from build123d import *

# Parameters (mm, degrees)
SKETCH_1_W                    = 120
SKETCH_1_H                    = 160
EXTRUDE_1_DEPTH               = 20
CHAMFER_1_SIZE                = 5
HOLE_WIZARD_M10_1_D           = 11
HOLE_WIZARD_M10_1_CBORE_D     = 18
HOLE_WIZARD_M10_1_CBORE_DEPTH = 10
CUT_EXTRUDE_1_REACH           = 103.98
SKETCH_6_R                    = 4


with BuildPart() as part:
    # 草圖1 → 伸長1 (new body)
    with BuildSketch(Plane(origin=(0, 0, 0), x_dir=(1, 0, 0), z_dir=(0, 1, 0))):
        Rectangle(SKETCH_1_W, SKETCH_1_H)
    extrude(amount=EXTRUDE_1_DEPTH)

    # 導角1
    chamfer_1_edges = [part.edges().sort_by_distance(p)[0] for p in [
        (-60, 10, -80),
        (60, 10, -80),
        (60, 10, 80),
        (-60, 10, 80),
    ]]
    chamfer(chamfer_1_edges, length=CHAMFER_1_SIZE)

    # M10 六角承窩頭蓋螺釘的柱孔1 (through all)
    with Locations(Plane(origin=(0, 20, 0), x_dir=(-1, 0, 0), z_dir=(0, 1, 0))):
        with Locations((40, -65.65), (40, -15.65), (40, 15.65), (40, 65.65), (-40, -65.65), (-40, -15.65), (-40, 15.65), (-40, 65.65)):
            CounterBoreHole(HOLE_WIZARD_M10_1_D / 2, HOLE_WIZARD_M10_1_CBORE_D / 2, HOLE_WIZARD_M10_1_CBORE_DEPTH)

    # 草圖6 → 除料-伸長1 (cut, up to next)
    with BuildSketch(Plane(origin=(0, 20, 0), x_dir=(1, 0, 0), z_dir=(0, 1, 0)), mode=Mode.PRIVATE) as cut_extrude_1_sk1:
        with Locations(Location((40, -40.65, 0), (0, 0, 270))):
            Circle(SKETCH_6_R)
    cut_extrude_1_tool1 = extrude(cut_extrude_1_sk1.sketch, amount=-CUT_EXTRUDE_1_REACH, mode=Mode.PRIVATE) & part.part
    # 草圖6 → 除料-伸長1 (cut, up to next)
    with BuildSketch(Plane(origin=(0, 20, 0), x_dir=(1, 0, 0), z_dir=(0, 1, 0)), mode=Mode.PRIVATE) as cut_extrude_1_sk2:
        with Locations(Location((-40, -40.65, 0), (0, 0, 270))):
            Circle(SKETCH_6_R)
    cut_extrude_1_tool2 = extrude(cut_extrude_1_sk2.sketch, amount=-CUT_EXTRUDE_1_REACH, mode=Mode.PRIVATE) & part.part
    # 草圖6 → 除料-伸長1 (cut, up to next)
    with BuildSketch(Plane(origin=(0, 20, 0), x_dir=(1, 0, 0), z_dir=(0, 1, 0)), mode=Mode.PRIVATE) as cut_extrude_1_sk3:
        with BuildLine():
            Line((39, 36.65), (41, 36.65))
            ThreePointArc((41, 36.65), (45, 40.65), (41, 44.65))
            Line((41, 44.65), (39, 44.65))
            ThreePointArc((39, 44.65), (35, 40.65), (39, 36.65))
        make_face()
    cut_extrude_1_tool3 = extrude(cut_extrude_1_sk3.sketch, amount=-CUT_EXTRUDE_1_REACH, mode=Mode.PRIVATE) & part.part
    # 草圖6 → 除料-伸長1 (cut, up to next)
    with BuildSketch(Plane(origin=(0, 20, 0), x_dir=(1, 0, 0), z_dir=(0, 1, 0)), mode=Mode.PRIVATE) as cut_extrude_1_sk4:
        with BuildLine():
            Line((-41, 36.65), (-39, 36.65))
            ThreePointArc((-39, 36.65), (-35, 40.65), (-39, 44.65))
            Line((-39, 44.65), (-41, 44.65))
            ThreePointArc((-41, 44.65), (-45, 40.65), (-41, 36.65))
        make_face()
    cut_extrude_1_tool4 = extrude(cut_extrude_1_sk4.sketch, amount=-CUT_EXTRUDE_1_REACH, mode=Mode.PRIVATE) & part.part
    add(cut_extrude_1_tool1.solids().sort_by_distance((40, 20, 40.65))[0], mode=Mode.SUBTRACT)
    add(cut_extrude_1_tool2.solids().sort_by_distance((-40, 20, 40.65))[0], mode=Mode.SUBTRACT)
    add(cut_extrude_1_tool3.solids().sort_by_distance((40, 20, -40.65))[0], mode=Mode.SUBTRACT)
    add(cut_extrude_1_tool4.solids().sort_by_distance((-40, 20, -40.65))[0], mode=Mode.SUBTRACT)


solid = part.part
The listing builds one solid part. Answer for the finished solid, in the listing's coordinates (mm). A direction names the side the tool comes from. Coordinates: 2 decimals unless noted, no trailing zeros. Order: outer loops, then holes, each group sorted by start corner. A loop starts at its lowest first (then second) coordinate and runs counter-clockwise, first axis right, second up. Notation, with made-up numbers: (56, -8.75) -> (67, -8.75) arc R14 ccw to (67, 13.25) -> close; hole circle Ø6 at (7.5, -40). An arc over 180 degrees is marked (long way). Answer in a Markdown table with one row per item. Add a question column.
Item 1: Find section D-D (z = -15.65). Write down the section's boundary in (x, y).
Item 2: Each of these flat-tipped pins is pushed along its axis until it touches: P1, Ø7, axis at x = 40, z = 40.65, coming from the +Y side; P2, Ø9, axis at x = -42, z = 63, coming from the +Y side. Where does it stop, or does it pass through?
Item 3: Find section B-B (y = 7.5). State how many separate pieces and enclosed holes the cut face has, then the cut area to 3 significant figures.
Item 4: Find the intervals of material crossed by L1, parallel to X at y = 4.25, z = -20; L2, parallel to X at y = 14, z = -42, in increasing order. Write a range as from..to.
Item 5: Determine the mould class of faces 4 (the face through (-1, 10, 80)), 5 (the face through (-1, 0, -1)), 6 (the face through (-45.495, 4.93, 65.892)) for opening direction Z: +Z half, -Z half, draft (parallel to the pull), parting line (faces both ways), or undercut.
Item 6: Find section C-C (z = 40.65). Write down the section's boundary in (x, y), then the cut area to 3 significant figures.
Item 7: Which of the six approach directions +Z, -Z, +X, -X, +Y, -Y give full straight-line access (tool end or side, diameter ignored) to faces 1 (the face through (-35, 10.1, -40.6)), 2 (the face through (-1, 20, -1)), 3 (the face through (-43.9, 10, -61.5))?
Item 8: Find section A-A (z = -40.65). Write down the section's boundary in (x, y).
Result set:
| question | item | result |
|---|---|---|
| 1 | outline | (-60, 0) -> (-45.5, 0) -> (-45.5, 10) -> (-49, 10) -> (-49, 20) -> (-60, 20) -> close; (-34.5, 0) -> (34.5, 0) -> (34.5, 10) -> (31, 10) -> (31, 20) -> (-31, 20) -> (-31, 10) -> (-34.5, 10) -> close; (45.5, 0) -> (60, 0) -> (60, 20) -> (49, 20) -> (49, 10) -> (45.5, 10) -> close |
| 2 | P1 | passes through |
| 2 | P2 | stops at y = 10 |
| 3 | separate pieces | 1 |
| 3 | enclosed holes | 12 |
| 3 | area | 18,200 mm² |
| 4 | L1 | x = -60..-43.37, -36.63..36.63, 43.37..60 |
| 4 | L2 | x = -60..-44.77, -35.23..35.23, 44.77..60 |
| 5 | face 4 | +Z half |
| 5 | face 5 | draft |
| 5 | face 6 | undercut |
| 6 | outline | (-60, 0) -> (-44, 0) -> (-44, 20) -> (-60, 20) -> close; (-36, 0) -> (36, 0) -> (36, 20) -> (-36, 20) -> close; (44, 0) -> (60, 0) -> (60, 20) -> (44, 20) -> close |
| 6 | area | 2,080 mm² |
| 7 | face 1 | +Y, -Y |
| 7 | face 2 | +Z, -Z, +X, -X, +Y |
| 7 | face 3 | +Y |
| 8 | outline | (-60, 0) -> (-45, 0) -> (-45, 20) -> (-60, 20) -> close; (-35, 0) -> (35, 0) -> (35, 20) -> (-35, 20) -> close; (45, 0) -> (60, 0) -> (60, 20) -> (45, 20) -> close |
